Part model, mm, in its own coordinate system. Face numbers are marked on the shaded views. A direction names the side the tool comes from. Give positions to 0.01 mm unless a question says otherwise; leave off trailing zeros. Write each loop counter-clockwise with the first axis right and the second up, starting at its lowest first coordinate (ties: lowest second). Pieces come first, ordered by that corner, then holes. Notation, with made-up numbers: M 53,44 L 65,44 A19 cw 65,55 Z; hole C -33.75,-15 d1. An arc over 180 degrees is marked long. Use CSV: the item, a comma, the result in double quotes. Start each with the question number.
1. Band-saw the part on D-D, the plane x = 149. List the corners of the cut face in (y, z).
2. 3-axis set-ups, long thin cutter, end or side, ignore diameter. For the marked faces 1, 2, 3 and 4: which of +Z, -Z, +X, -X, +Y, -Y reach the whole face in a straight line?
3. Band-saw the part on B-B, the plane y = 88. List the corners of the cut face in (x, z), then the cut area to 3 significant figures.
4. Drill centre lines: line 1 along Z through (x, y) = (50, 28); line 2 along X through (y, z) = (112.5, -67.5); line 3 along X through (y, z) = (65.5, -65.5). Where is each one in solid material? Low to high. Write a range as from..to.
5. Band-saw the part on A-A, the plane x = 92.5. List the corners of the cut face in (y, z).
6. Mould opens along Z. For the marked faces 5, 6 and 7 say: pulls with the +Z half, pulls with the -Z half, needs draft (parallel to the pull), parting line crosses it, or undercut.
7. Drop flat-ended pins along their axis: pin 1 Ø16 at (y, z) = (6, -88) entering from -X; pin 2 Ø10 at (x, y) = (146.5, 29.5) entering from -Z; pin 3 Ø12 at (x, y) = (33, 15) entering from -Z; pin 4 Ø10 at (x, z) = (85.5, -102.5) entering from -Y. Give the stop position or say it passes through.
8. Band-saw the part on C-C, the plane z = -85. List the corners of the cut face in (x, y), then the cut area to 3 significant figures.
from build123d import *

# Parameters (mm, degrees)
SKETCH1_W           = 180
SKETCH1_H           = 120
BOSS_EXTRUDE2_DEPTH = 120
SKETCH2_W           = 110
SKETCH2_H           = 10
CUT_EXTRUDE1_DEPTH  = 120
CUT_EXTRUDE2_DEPTH  = 120
CUT_EXTRUDE3_DEPTH  = 120
CUT_EXTRUDE4_DEPTH  = 120
SKETCH6_R           = 5
CUT_EXTRUDE5_DEPTH  = 120
SKETCH7_R           = 10
CUT_EXTRUDE6_DEPTH  = 120
CUT_EXTRUDE7_DEPTH  = 30
BOSS_EXTRUDE3_DEPTH = 30
CUT_EXTRUDE8_DEPTH  = 60
CUT_EXTRUDE9_DEPTH  = 60
CUT_EXTRUDE10_DEPTH = 60
CUT_EXTRUDE11_DEPTH = 60
SKETCH15_W          = 25
SKETCH15_H          = 5
BOSS_EXTRUDE5_DEPTH = 29.999
SKETCH16_R          = 10
CUT_EXTRUDE12_DEPTH = 125.999
SKETCH17_R          = 20
SKETCH17_R_2        = 10
CUT_EXTRUDE13_DEPTH = 30
SKETCH19_R          = 10
SKETCH19_R_2        = 5
CUT_EXTRUDE14_DEPTH = 20
SKETCH20_R          = 20
SKETCH20_R_2        = 10
CUT_EXTRUDE15_DEPTH = 84.461973219
BOSS_EXTRUDE6_DEPTH = 20
BOSS_EXTRUDE7_DEPTH = 20


with BuildPart() as part:
    # Sketch1 → Boss-Extrude2 (new body)
    with BuildSketch(Plane(origin=(0, 0, 0), x_dir=(1, 0, 0), z_dir=(0, 1, 0))):
        with Locations((90, 60)):
            Rectangle(SKETCH1_W, SKETCH1_H)
    extrude(amount=BOSS_EXTRUDE2_DEPTH)

    # Sketch2 → Cut-Extrude1 (cut)
    with BuildSketch(Plane(origin=(0, 0, 0), x_dir=(1, 0, 0), z_dir=(0, 1, 0))):
        with Locations((55, 115)):
            Rectangle(SKETCH2_W, SKETCH2_H)
        with Locations((55, 5)):
            Rectangle(SKETCH2_W, SKETCH2_H)
    extrude(amount=CUT_EXTRUDE1_DEPTH, mode=Mode.SUBTRACT)

    # Sketch3 → Cut-Extrude2 (cut)
    with BuildSketch(Plane(origin=(0, 120, 0), x_dir=(1, 0, 0), z_dir=(0, 1, 0))):
        with BuildLine():
            Line((110, 110), (110, 120))
            Line((110, 120), (120, 120))
            ThreePointArc((120, 120), (117.071067812, 112.928932188), (110, 110))
        make_face()
        with BuildLine():
            Line((120, 0), (110, 0))
            Line((110, 0), (110, 10))
            ThreePointArc((110, 10), (117.071067812, 7.071067812), (120, 0))
        make_face()
    extrude(amount=-CUT_EXTRUDE2_DEPTH, mode=Mode.SUBTRACT)

    # Sketch4 → Cut-Extrude3 (cut)
    with BuildSketch(Plane(origin=(0, 120, 0), x_dir=(1, 0, 0), z_dir=(0, 1, 0))):
        with BuildLine():
            Line((180, 120), (120, 120))
            ThreePointArc((120, 120), (162.426406871, 102.426406871), (180, 60))
            Line((180, 60), (180, 120))
        make_face()
        with BuildLine():
            Line((180, 0), (180, 60))
            ThreePointArc((180, 60), (162.426406871, 17.573593129), (120, 0))
            Line((120, 0), (180, 0))
        make_face()
    extrude(amount=-CUT_EXTRUDE3_DEPTH, mode=Mode.SUBTRACT)

    # Sketch5 → Cut-Extrude4 (cut)
    with BuildSketch(Plane(origin=(0, 120, 0), x_dir=(1, 0, 0), z_dir=(0, 1, 0))):
        with BuildLine():
            ThreePointArc((0, 59.999999737), (14.644660848, 95.355338966), (50, 110))
            Line((50, 110), (0, 110))
            Line((0, 110), (0, 59.999999737))
        make_face()
        with BuildLine():
            ThreePointArc((50, 10), (14.644661034, 24.644660848), (0, 59.999999737))
            Line((0, 59.999999737), (0, 10))
            Line((0, 10), (50, 10))
        make_face()
    extrude(amount=-CUT_EXTRUDE4_DEPTH, mode=Mode.SUBTRACT)

    # Sketch6 → Cut-Extrude5 (cut)
    with BuildSketch(Plane(origin=(0, 120, 0), x_dir=(1, 0, 0), z_dir=(0, 1, 0))):
        with Locations((25, 85)):
            Circle(SKETCH6_R)
        with Locations((25, 35)):
            Circle(SKETCH6_R)
    extrude(amount=-CUT_EXTRUDE5_DEPTH, mode=Mode.SUBTRACT)

    # Sketch7 → Cut-Extrude6 (cut)
    with BuildSketch(Plane(origin=(0, 120, 0), x_dir=(1, 0, 0), z_dir=(0, 1, 0))):
        with Locations((120, 60)):
            Circle(SKETCH7_R)
    extrude(amount=-CUT_EXTRUDE6_DEPTH, mode=Mode.SUBTRACT)

    # Sketch9 → Cut-Extrude7 (cut)
    with BuildSketch(Plane(origin=(0, 120, 0), x_dir=(1, 0, 0), z_dir=(0, 1, 0))):
        with BuildLine():
            Line((120, 120), (120, 0))
            ThreePointArc((120, 0), (117.071067812, 7.071067812), (110, 10))
            Line((110, 10), (50, 10))
            ThreePointArc((50, 10), (0, 60), (50, 110))
            Line((50, 110), (110, 110))
            ThreePointArc((110, 110), (117.071067812, 112.928932188), (120, 120))
        make_face()
    extrude(amount=-CUT_EXTRUDE7_DEPTH, mode=Mode.SUBTRACT)

    # Sketch10 → Boss-Extrude3 (add)
    with BuildSketch(Plane(origin=(0, 90, 0), x_dir=(1, 0, 0), z_dir=(0, 1, 0))):
        with BuildLine():
            Line((120, 70), (120, 80))
            ThreePointArc((120, 80), (100, 60), (120, 40))
            Line((120, 40), (120, 50))
            ThreePointArc((120, 50), (110, 60), (120, 70))
        make_face()
    extrude(amount=BOSS_EXTRUDE3_DEPTH)

    # Sketch11 → Cut-Extrude8 (cut)
    with BuildSketch(Plane(origin=(0, 120, 0), x_dir=(1, 0, 0), z_dir=(0, 1, 0))):
        with BuildLine():
            Line((124.743133772, 80), (124.743133772, 110))
            ThreePointArc((124.743133772, 110), (158.684259269, 95.941125497), (172.743133772, 62))
            Line((172.743133772, 62), (142.743133772, 62))
            ThreePointArc((142.743133772, 62), (137.471055833, 74.727922061), (124.743133772, 80))
        make_face()
    extrude(amount=-CUT_EXTRUDE8_DEPTH, mode=Mode.SUBTRACT)

    # Sketch12 → Cut-Extrude9 (cut)
    with BuildSketch(Plane(origin=(0, 120, 0), x_dir=(1, 0, 0), z_dir=(0, 1, 0))):
        with BuildLine():
            Line((124.743133772, 39.722678499), (124.743133772, 9.722678499))
            ThreePointArc((124.743133772, 9.722678499), (158.684259269, 23.781553002), (172.743133772, 57.722678499))
            Line((172.743133772, 57.722678499), (142.743133772, 57.722678499))
            ThreePointArc((142.743133772, 57.722678499), (137.471055833, 44.994756437), (124.743133772, 39.722678499))
        make_face()
    extrude(amount=-CUT_EXTRUDE9_DEPTH, mode=Mode.SUBTRACT)

    # Sketch13 → Cut-Extrude10 (cut)
    with BuildSketch(Plane(origin=(0, 60, 0), x_dir=(1, 0, 0), z_dir=(0, 1, 0))):
        with BuildLine():
            Line((124.743133772, 80), (124.743133772, 100))
            ThreePointArc((124.743133772, 100), (151.613191457, 88.870057685), (162.743133772, 62))
            Line((162.743133772, 62), (142.743133772, 62))
            ThreePointArc((142.743133772, 62), (137.471055833, 74.727922061), (124.743133772, 80))
        make_face()
    extrude(amount=-CUT_EXTRUDE10_DEPTH, mode=Mode.SUBTRACT)

    # Sketch14 → Cut-Extrude11 (cut)
    with BuildSketch(Plane(origin=(0, 60, 0), x_dir=(1, 0, 0), z_dir=(0, 1, 0))):
        with BuildLine():
            Line((124.743133772, 39.722678499), (124.743133772, 19.722678499))
            ThreePointArc((124.743133772, 19.722678499), (151.613191457, 30.852620814), (162.743133772, 57.722678499))
            Line((162.743133772, 57.722678499), (142.743133772, 57.722678499))
            ThreePointArc((142.743133772, 57.722678499), (137.471055833, 44.994756437), (124.743133772, 39.722678499))
        make_face()
    extrude(amount=-CUT_EXTRUDE11_DEPTH, mode=Mode.SUBTRACT)

    # Sketch15 → Boss-Extrude5 (add)
    with BuildSketch(Plane(origin=(0, 90, 0), x_dir=(1, 0, 0), z_dir=(0, 1, 0))):
        with Locations((87.656865167, 60)):
            Rectangle(SKETCH15_W, SKETCH15_H)
    extrude(amount=BOSS_EXTRUDE5_DEPTH)

    # Sketch16 → Cut-Extrude12 (cut)
    with BuildSketch(Plane(origin=(0, 90, 0), x_dir=(1, 0, 0), z_dir=(0, 1, 0))):
        with Locations((50, 60)):
            Circle(SKETCH16_R)
    extrude(amount=-CUT_EXTRUDE12_DEPTH, mode=Mode.SUBTRACT)

    # Sketch17 → Cut-Extrude13 (cut)
    with BuildSketch(Plane(origin=(0, 90, 0), x_dir=(1, 0, 0), z_dir=(0, 1, 0))):
        with Locations((50, 60)):
            Circle(SKETCH17_R)
        with Locations((50, 60)):
            Circle(SKETCH17_R_2, mode=Mode.SUBTRACT)
    extrude(amount=-CUT_EXTRUDE13_DEPTH, mode=Mode.SUBTRACT)

    # Sketch19 → Cut-Extrude14 (cut)
    with BuildSketch(Plane(origin=(0, 0, 0), x_dir=(-1, 0, 0), z_dir=(0, -1, 0))):
        with Locations((-50, 60)):
            Circle(SKETCH19_R)
        with BuildLine():
            Line((-50, 110), (-50, 10))
            ThreePointArc((-50, 10), (0, 60), (-50, 110))
        make_face()
        with Locations((-25, 35)):
            Circle(SKETCH19_R_2, mode=Mode.SUBTRACT)
        with Locations((-25, 85)):
            Circle(SKETCH19_R_2, mode=Mode.SUBTRACT)
    extrude(amount=-CUT_EXTRUDE14_DEPTH, mode=Mode.SUBTRACT)

    # Sketch20 → Cut-Extrude15 (cut)
    with BuildSketch(Plane(origin=(0, 60, 0), x_dir=(1, 0, 0), z_dir=(0, 1, 0))):
        with Locations((50, 60)):
            Circle(SKETCH20_R)
        with Locations((50, 60)):
            Circle(SKETCH20_R_2, mode=Mode.SUBTRACT)
    extrude(amount=-CUT_EXTRUDE15_DEPTH, mode=Mode.SUBTRACT)

    # Sketch21 → Boss-Extrude6 (add)
    with BuildSketch(Plane.XZ.offset(-20)):
        with BuildLine():
            Line((50, -70), (50, -80))
            ThreePointArc((50, -80), (30, -60), (50, -40))
            Line((50, -40), (50, -50))
            ThreePointArc((50, -50), (40, -60), (50, -70))
        make_face()
    extrude(amount=-BOSS_EXTRUDE6_DEPTH)

    # Sketch22 → Boss-Extrude7 (add)
    with BuildSketch(Plane.XZ.offset(-20)):
        with BuildLine():
            Line((50, -70), (50, -80))
            ThreePointArc((50, -80), (70, -60), (50, -40))
            Line((50, -40), (50, -50))
            ThreePointArc((50, -50), (60, -60), (50, -70))
        make_face()
    extrude(amount=-BOSS_EXTRUDE7_DEPTH)


solid = part.part
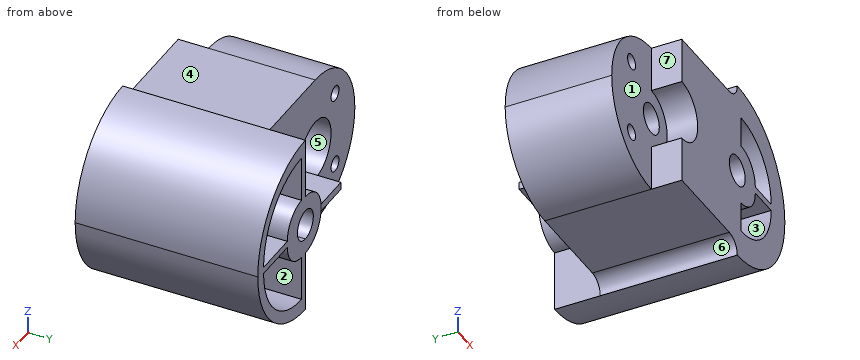
Output:
1,outline,"M 0,-112.53 L 120,-112.53 L 120,-103.42 L 60,-103.42 L 60,-91.25 L 0,-91.25 Z; M 0,-62 L 120,-62 L 120,-57.72 L 0,-57.72 Z; M 0,-28.47 L 60,-28.47 L 60,-16.3 L 120,-16.3 L 120,-7.47 L 0,-7.47 Z"
2,face 1,"-X, -Y"
2,face 2,"+Y"
2,face 3,"+Y, -Y"
2,face 4,"+Z, -X, +Y, -Y"
3,outline,"M 50,-110 L 110,-110 A10 cw 120,-120 A60 ccw 120,0 A10 cw 110,-10 L 50,-10 A50 ccw Z; hole C 25,-85 d10; hole C 25,-35 d10; hole C 50,-60 d40; hole C 120,-60 d20; hole M 124.74,-110 A48 ccw 172.74,-62 L 142.74,-62 A18 cw 124.74,-80 Z; hole M 124.74,-39.72 A18 cw 142.74,-57.72 L 172.74,-57.72 A48 ccw 124.74,-9.72 Z"
3,area,"11,800 mm²"
4,line 1,"z = -110..-70, -50..-10"
4,line 2,"x = 101.46..113.39, 126.61..141.88, 172.43..179.53"
4,line 3,"x = 0.3..30.77, 69.23..111.65, 128.35..142.4, 172.62..179.75"
5,outline,"M 0,-110 L 90,-110 L 90,-62.5 L 120,-62.5 L 120,-57.5 L 90,-57.5 L 90,-10 L 0,-10 Z"
6,face 5,"undercut"
6,face 6,"pulls with the -Z half"
6,face 7,"needs draft"
7,pin 1,"stops at x = 50"
7,pin 2,"stops at z = -116.02"
7,pin 3,"stops at z = -108.09"
7,pin 4,"stops at y = 0"
8,outline,"M 6.7,20 L 20,20 L 20,90 L 6.7,90 Z; M 30,20 L 50,20 L 50,0 L 124.74,0 L 124.74,120 L 120,120 L 120,90 L 30,90 Z; M 154.99,0 L 174.54,0 L 174.54,120 L 166.87,120 L 166.87,60 L 154.99,60 Z"
8,area,"10,800 mm²"
